Geometry: final body of the model. Coordinates: model frame, mm. A direction names the side the tool comes from. Give positions to 0.01 mm unless a question says otherwise; leave off trailing zeros. Write each loop counter-clockwise with the first axis right and the second up, starting at its lowest first coordinate (ties: lowest second). Pieces come first, ordered by that corner, then holes. Notation, with made-up numbers: (-39, 70) - (18, 70) arc R14 cw to (18, 83) - close; hole circle Ø5 at (-29.75, 60). An arc over 180 degrees is marked (long way). Return JSON: item names as keys, results as strings.
from build123d import *

# Parameters (mm, degrees)
BOSS_EXTRUDE1_DEPTH        = 6
F_7_0_7_DIAMETER_HOLE1_D   = 7
LPATTERN1_COUNT            = 4
LPATTERN1_PITCH            = 22
FILLET1_R                  = 5
MIRROR1_COPY_1_D           = 7
MIRROR1_COPY_2_D           = 7
MIRROR1_COPY_3_D           = 7
FILLET1_OF_MIRROR1_R       = 5
MIRROR5_COPY_1_D           = 7
MIRROR5_COPY_2_D           = 7
MIRROR5_COPY_3_D           = 7
FILLET1_OF_MIRROR5_R       = 5
MIRROR6_START              = -6
MIRROR6_OUTLINE_R          = 3.5
MIRROR6_DEPTH              = 12
F_6_8_6_8_DIAMETER_HOLE1_D = 6.8
SKETCH9_W                  = 314.382892994
SKETCH9_H                  = 141.517755545
CUT_EXTRUDE1_DEPTH         = 196.624640575


# Read off the part's stored shape, not the designer's step: Mirror6
with BuildPart() as part:
    # Sketch1 → Boss-Extrude1 (new, symmetric)
    with BuildSketch(Plane.XY):
        with BuildLine():
            Line((0, 0), (0, 125))
            Line((0, 125), (34, 125))
            ThreePointArc((34, 125), (61.824855787, 57.824855787), (129, 30))
            Line((129, 30), (150, 30))
            Line((150, 30), (150, 0))
            Line((150, 0), (114.303256495, 0))
            Line((114.303256495, 0), (0, 0))
        make_face()
    boss_extrude1 = extrude(amount=BOSS_EXTRUDE1_DEPTH, both=True)

    # Ø7.0 (7) Diameter Hole1 (through all)
    with Locations(Plane.XY.offset(6)):
        with Locations((26, 110)):
            f_7_0_7_diameter_hole1 = Hole(F_7_0_7_DIAMETER_HOLE1_D / 2)

    # LPattern1: Ø7.0 (7) Diameter Hole1 ×4
    with Locations(*[(0, -i * LPATTERN1_PITCH, 0) for i in range(1, LPATTERN1_COUNT)]):
        add(f_7_0_7_diameter_hole1, mode=Mode.SUBTRACT)

    # Fillet1
    fillet1_edges = [part.edges().sort_by_distance(p)[0] for p in [
        (34, 125, 0),
        (150, 30, 0),
    ]]
    fillet(fillet1_edges, radius=FILLET1_R)

    # Mirror1: Boss-Extrude1, Ø7.0 (7) Diameter Hole1 across plane
    add(boss_extrude1.mirror(Plane(origin=(0, 0, 6), x_dir=(0, 0, 1), z_dir=(1, 0, 0))))
    add(f_7_0_7_diameter_hole1.mirror(Plane(origin=(0, 0, 6), x_dir=(0, 0, 1), z_dir=(1, 0, 0))), mode=Mode.SUBTRACT)

    # Mirror1 copy 1 (through all)
    with Locations(Plane(origin=(0, -22, 6), x_dir=(-1, 0, 0), z_dir=(0, 0, 1))):
        with Locations((26, -110)):
            Hole(MIRROR1_COPY_1_D / 2)

    # Mirror1 copy 2 (through all)
    with Locations(Plane(origin=(0, -44, 6), x_dir=(-1, 0, 0), z_dir=(0, 0, 1))):
        with Locations((26, -110)):
            Hole(MIRROR1_COPY_2_D / 2)

    # Mirror1 copy 3 (through all)
    with Locations(Plane(origin=(0, -66, 6), x_dir=(-1, 0, 0), z_dir=(0, 0, 1))):
        with Locations((26, -110)):
            Hole(MIRROR1_COPY_3_D / 2)

    # Fillet1 of Mirror1
    fillet1_of_mirror1_edges = [part.edges().sort_by_distance(p)[0] for p in [
        (-34, 125, 0),
        (-150, 30, 0),
    ]]
    fillet(fillet1_of_mirror1_edges, radius=FILLET1_OF_MIRROR1_R)

    # Mirror5: Boss-Extrude1, Ø7.0 (7) Diameter Hole1 across plane
    add(boss_extrude1.mirror(Plane.ZX))
    add(f_7_0_7_diameter_hole1.mirror(Plane.ZX), mode=Mode.SUBTRACT)

    # Mirror5 copy 1 (through all)
    with Locations(Plane(origin=(0, 22, 6), x_dir=(1, 0, 0), z_dir=(0, 0, 1))):
        with Locations((26, -110)):
            Hole(MIRROR5_COPY_1_D / 2)

    # Mirror5 copy 2 (through all)
    with Locations(Plane(origin=(0, 44, 6), x_dir=(1, 0, 0), z_dir=(0, 0, 1))):
        with Locations((26, -110)):
            Hole(MIRROR5_COPY_2_D / 2)

    # Mirror5 copy 3 (through all)
    with Locations(Plane(origin=(0, 66, 6), x_dir=(1, 0, 0), z_dir=(0, 0, 1))):
        with Locations((26, -110)):
            Hole(MIRROR5_COPY_3_D / 2)

    # Fillet1 of Mirror5
    fillet1_of_mirror5_edges = [part.edges().sort_by_distance(p)[0] for p in [
        (34, -125, 0),
        (150, -30, 0),
    ]]
    fillet(fillet1_of_mirror5_edges, radius=FILLET1_OF_MIRROR5_R)

    # Mirror6 outline → Mirror6 (add)
    with BuildSketch(Plane.XY.offset(MIRROR6_START)):
        with BuildLine():
            Line((0, 0), (-150, 0))
            Line((-150, 0), (-150, -25))
            ThreePointArc((-150, -25), (-148.535533906, -28.535533906), (-145, -30))
            Line((-145, -30), (-129, -30))
            ThreePointArc((-129, -30), (-63.525768428, -56.165960456), (-34.118824312, -120.25))
            ThreePointArc((-34.118824312, -120.25), (-32.571090411, -123.622844187), (-29.125078223, -125))
            Line((-29.125078223, -125), (0, -125))
            Line((0, -125), (0, 0))
        make_face()
        with Locations((-26, -110)):
            Circle(MIRROR6_OUTLINE_R, mode=Mode.SUBTRACT)
        with Locations((-26, -88)):
            Circle(MIRROR6_OUTLINE_R, mode=Mode.SUBTRACT)
        with Locations((-26, -66)):
            Circle(MIRROR6_OUTLINE_R, mode=Mode.SUBTRACT)
        with Locations((-26, -44)):
            Circle(MIRROR6_OUTLINE_R, mode=Mode.SUBTRACT)
    extrude(amount=MIRROR6_DEPTH)

    # Ø6.8 (6.8) Diameter Hole1 (through all)
    with Locations(Plane.XY.offset(6)):
        with Locations((130, 15), (100, 15), (70, 15), (115, -15), (85, -15), (55, -15)):
            f_6_8_6_8_diameter_hole1 = Hole(F_6_8_6_8_DIAMETER_HOLE1_D / 2)

    # Mirror7: Ø6.8 (6.8) Diameter Hole1 across plane
    add(f_6_8_6_8_diameter_hole1.mirror(Plane(origin=(0, 0, 0), x_dir=(0, 0, 1), z_dir=(1, 0, 0))), mode=Mode.SUBTRACT)

    # Sketch9 → Cut-Extrude1 (cut, through all)
    with BuildSketch(Plane.XY.offset(6)):
        with Locations((3.183624233, -100.758877772)):
            Rectangle(SKETCH9_W, SKETCH9_H)
    extrude(amount=-CUT_EXTRUDE1_DEPTH, mode=Mode.SUBTRACT)


solid = part.part
Q1. Set-up query: faces 1 (the flat face through (-137, 30, 0)), 2 (the cylindrical face through (51.86, -16.3, -0.08)). Return all of +Z, -Z, +X, -X, +Y, -Y with unobstructed straight access to the full face (end or side cutting, diameter ignored); none if empty.
Answer key:
{"face 1": "+Z, -Z, -X, +Y", "face 2": "+Z, -Z"}
Q2. Section query C-C, the plane z = -3.75. Count the separate pieces of the cut face and the enclosed holes in it, plus the area to 3 significant figures.
Answer key:
{"separate pieces": "1", "enclosed holes": "20", "area": "27,600 mm^2"}
Q3. Material intervals for probe 1 along Y at (x, z) = (-26, 1); probe 2 along Y at (x, z) = (-27, 5.75); probe 3 along Y at (x, z) = (114, 2), sorted ascending. Write a range as [from, to].
Answer key:
{"probe 1": "y = [-30, 40.5], [47.5, 62.5], [69.5, 84.5], [91.5, 106.5], [113.5, 125]", "probe 2": "y = [-30, 40.65], [47.35, 62.65], [69.35, 84.65], [91.35, 106.65], [113.35, 125]", "probe 3": "y = [-30, -18.25], [-11.75, 31.19]"}
Q4. Mould query, pull axis X, two halves, no side actions, for faces 3 (the flat face through (-150, 0, 0)), 4 (the flat face through (137, 30, 0)), 5 (the cylindrical face through (62.797, 56.867, 0.084)), 6 (the cylindrical face through (-66.86, 13.7, -0.08)). Classes: pulls with the +X half, pulls with the -X half, needs draft (parallel to the pull), parting line crosses it, or undercut.
Answer key:
{"face 3": "pulls with the -X half", "face 4": "needs draft", "face 5": "pulls with the +X half", "face 6": "undercut"}
Q5. Section query D-D, the plane x = -100. Return the cut outline in (y, z), plus the area to 3 significant figures.
Answer key:
{"outline": "(-30, -6) - (11.6, -6) - (11.6, 6) - (-30, 6) - close; (18.4, -6) - (34.53, -6) - (34.53, 6) - (18.4, 6) - close", "area": "693 mm^2"}
Q6. Pin query (flat end, axial travel): P1, Ø6, axis at x = -137.5, z = 0.5, coming from the +Y side; P2, Ø6, axis at x = -130, y = 15, coming from the +Z side; P3, Ø1, axis at x = 60, z = -2.5, coming from the +Y side; P4, Ø11, axis at x = -100, y = 15, coming from the +Z side. Return the tip coordinate at first contact, or that it passes through.
Answer key:
{"P1": "stops at y = 30", "P2": "passes through", "P3": "stops at y = 60.23", "P4": "stops at z = 6"}
Q7. Section query B-B, the plane y = 15. Return the cut outline in (x, z).
Answer key:
{"outline": "(-150, -6) - (-133.4, -6) - (-133.4, 6) - (-150, 6) - close; (-126.6, -6) - (-103.4, -6) - (-103.4, 6) - (-126.6, 6) - close; (-96.6, -6) - (-73.4, -6) - (-73.4, 6) - (-96.6, 6) - close; (-66.6, -6) - (66.6, -6) - (66.6, 6) - (-66.6, 6) - close; (73.4, -6) - (96.6, -6) - (96.6, 6) - (73.4, 6) - close; (103.4, -6) - (126.6, -6) - (126.6, 6) - (103.4, 6) - close; (133.4, -6) - (150, -6) - (150, 6) - (133.4, 6) - close"}
Q8. Section query A-A, the plane x = 26. Return the cut outline in (y, z).
Answer key:
{"outline": "(-30, -6) - (40.5, -6) - (40.5, 6) - (-30, 6) - close; (47.5, -6) - (62.5, -6) - (62.5, 6) - (47.5, 6) - close; (69.5, -6) - (84.5, -6) - (84.5, 6) - (69.5, 6) - close; (91.5, -6) - (106.5, -6) - (106.5, 6) - (91.5, 6) - close; (113.5, -6) - (125, -6) - (125, 6) - (113.5, 6) - close"}
